Check sheet for the modelled part. Datum: model origin and axes. Units: mm. Give positions to 0.01 mm unless a question says otherwise; leave off trailing zeros. Loops run counter-clockwise (first coordinate to the right, second up) from the corner with the lowest first, then second, coordinate; pieces in that order, holes last. Notation, with made-up numbers: (2, 35) - (43, 35) arc R25 ccw to (43, 56) - close; hole circle Ø3 at (-7.75, 30.25). An arc over 180 degrees is marked (long way). Answer in a Markdown table with one row per item. Add a question column.
(1) Go/stop test with flat-tipped pins: P1, Ø3.5, axis at x = -18, z = 4, coming from the -Y side; P2, Ø2.5, axis at x = 17.73, y = -39, coming from the -Z side; P3, Ø1.5, axis at y = -22.5, z = 1, coming from the -X side. Record where each tip stops, or that it passes through.
(2) Thickness scan on L1, parallel to X at y = -37, z = 3.5; L2, parallel to X at y = -5, z = 5; L3, parallel to X at y = 34, z = 3.25. Record the ranges inside material, lowest first.
(3) Sectioned sample at C-C on x = -44.5. Enter the section's corners in (y, z).
(4) Sectioned sample at B-B on z = 4.75. State how many separate pieces and enclosed holes the cut face has, then the cut area to 3 significant figures.
(5) Sectioned sample at D-D on x = -0.5. Enter the section's corners in (y, z), then the cut area to 3 significant figures.
(6) Sectioned sample at A-A on y = 23. Enter the section's corners in (x, z).
from build123d import *

# Parameters (mm, degrees)
F0_W     = 8
F0_H     = 6
F0_H_2   = 5.6374937892
F0_W_2   = 4
F0_H_3   = 23
F0_W_3   = 38.2781559229
F0_H_4   = 34.3460934982
F1_DEPTH = 7
F2_D     = 2
F3_D     = 5.75


with BuildPart() as f1:
    # F0 (on Top) → F1 (new body)
    with BuildSketch(Plane.XY):
        Polygon((10.5, -45), (22.5, -45), (22.5, -10.6539065018), (22.5, 17.153987661), (0, 45), (-14.5, 45), (-14.5, 39), (-14.5, 16), (-14.5, 10.3625062108), (-22.5, 10.3625062108), (-22.5, -42.25), (-10.5080957781, -42.25), (-10.6281967604, -1.0001864958), (10.3717142302, -0.9390441602), align=None)
        Polygon((0, 45), (22.5, 17.153987661), (22.5, 45), align=None)
        Polygon((-30.5, 39), (-30.5, 45), (-55.0723059862, 45), (-55.0723059862, 10.3625062108), (-30.5, 10.3625062108), (-30.5, 16), align=None)
        with Locations((-26.5, 42)):
            Rectangle(F0_W, F0_H)
        Polygon((-14.5, 39), (-14.5, 45), (-22.5, 45), (-22.5, 39), (-18.5, 39), align=None)
        Polygon((-22.5, 16), (-22.5, 10.3625062108), (-14.5, 10.3625062108), (-14.5, 16), (-18.5, 16), align=None)
        with Locations((-26.5, 13.1812531054)):
            Rectangle(F0_W, F0_H_2)
        Polygon((22.5, 17.153987661), (22.5, -10.6539065018), (60.7781559229, -10.6539065018), (60.7781559229, 45), (22.5, 45), align=None)
        Polygon((0, 45), (22.5, 45), (60.7781559229, 45), (60.6384575367, 56.7700602114), (-55.0723059862, 56.7700602114), (-55.0723059862, 45), (-30.5, 45), (-22.5, 45), (-14.5, 45), align=None)
        with Locations((-16.5, 27.5)):
            Rectangle(F0_W_2, F0_H_3)
        with Locations((41.6390779614, -27.8269532509)):
            Rectangle(F0_W_3, F0_H_4)
    extrude(amount=F1_DEPTH)

    # F2 (through all)
    with Locations(Plane(origin=(0, 0, 0), x_dir=(1, 0, 0), z_dir=(0, 0, -1))):
        with Locations((-17.0669870824, 5), (-17.7734121563, 37), (17.7265878437, 39), (17.9330129176, 7)):
            Hole(F2_D / 2)

    # F3 (through all)
    with Locations(Plane(origin=(0, 0, 0), x_dir=(1, 0, 0), z_dir=(0, 0, -1))):
        with Locations((-10.5364832571, 32.5000529818), (10.4634277335, 32.4389106462)):
            Hole(F3_D / 2)


solid = f1.part
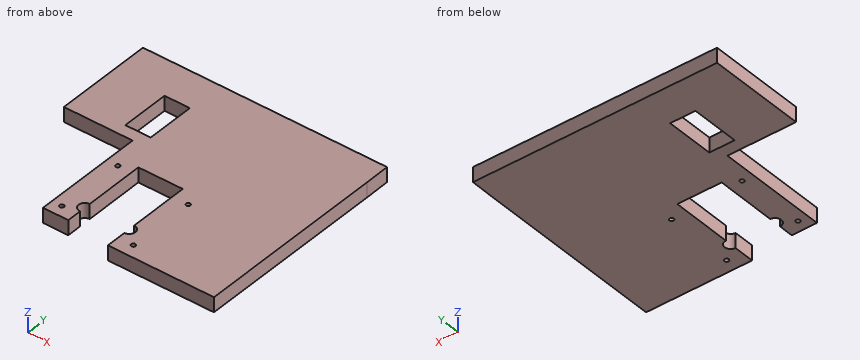
Reply:
| question | item | result |
|---|---|---|
| 1 | P1 | y = -42.25 |
| 1 | P2 | z = 0 |
| 1 | P3 | x = -22.5 |
| 2 | L1 | -22.5 to -18.77, -16.77 to -10.52, 10.48 to 60.78 |
| 2 | L2 | -22.5 to -18.07, -16.07 to -10.62, 10.38 to 60.78 |
| 2 | L3 | -55.07 to -30.5, -18.5 to 60.78 |
| 3 | outline | (10.36, 0) - (56.77, 0) - (56.77, 7) - (10.36, 7) - close |
| 4 | separate pieces | 1 |
| 4 | enclosed holes | 5 |
| 4 | area | 8,710 mm^2 |
| 5 | outline | (-0.97, 0) - (56.77, 0) - (56.77, 7) - (-0.97, 7) - close |
| 5 | area | 404 mm^2 |
| 6 | outline | (-55.07, 0) - (-30.5, 0) - (-30.5, 7) - (-55.07, 7) - close; (-18.5, 0) - (60.78, 0) - (60.78, 7) - (-18.5, 7) - close |
